Here's how the part is built. I have some questions about the finished solid (model axes, mm). Give positions to 0.01 mm unless a question says otherwise; leave off trailing zeros. Loops run counter-clockwise (first coordinate to the right, second up) from the corner with the lowest first, then second, coordinate; pieces in that order, holes last. Notation, with made-up numbers: (77.25, 30) - (134.25, 30) arc R27 cw to (134.25, 56) - close; hole circle Ø6 at (49.25, 76.25). An arc over 180 degrees is marked (long way). Use a Markdown table: item, result.
Autodesk Inventor part; units mm, degrees
ref_plane "YZ Plane" through (0, 0, 0) normal (1, 0, 0) x (0, 1, 0)
ref_plane "XZ Plane" through (0, 0, 0) normal (0, 1, 0) x (-1, 0, 0)
ref_plane "XY Plane" through (0, 0, 0) normal (0, 0, 1) x (1, 0, 0)
sketch "Sketch1" plane through (0, 0, 0) normal (0, 0, 1) x (1, 0, 0)
  line L0 (0, 0) -> (49.2125, 0)
  arc A0 (69.2791, -9.8278) -> (49.2125, 0) centre (49.2125, -25.4) ccw
  line L1 (69.2791, -9.8278) -> (116.6499, -70.8709)
  arc A1 (113.4684, -97.4512) -> (116.6499, -70.8709) centre (101.6, -82.55) ccw
  line L2 (113.4684, -97.4512) -> (70.102, -131.9913)
  arc A2 (48.0501, -139.7) -> (70.102, -131.9913) centre (48.0501, -104.3043) ccw
  line L3 (48.0501, -139.7) -> (0, -139.7)
  line L4 (0, -139.7) -> (0, 0)
  line L5 (0, -139.7) -> (12.7, -139.7) construction
  circle A3 centre (101.6, -82.55) radius 16 construction
  circle A4 centre (48.0501, -104.3043) radius 7.025 construction
  arc A5 (33.057, -35.4) -> (32.0953, -33.6463) centre (49.2125, -25.4) ccw construction
  circle A6 centre (38.1, -63.5) radius 17.907 construction
  circle A7 centre (71.7198, -40.8503) radius 7.025 construction
  circle A8 centre (38.1, -63.5) radius 19.05
  circle A9 centre (48.0501, -104.3043) radius 3
  circle A10 centre (101.6, -82.55) radius 9.525
  dimension "d0" = 19.05
  dimension "d1" = 38.1
  dimension "d4" = 6
  dimension "d5" = 19.05
extrude "Extrusion1" add sketch "Sketch1" along normal blind 6.35 contours L0 A0 L1 A1 L2 A2 L3 L4 | A8
chamfer "Chamfer1" distance 3.175 angle 45 7 edges at (92.9645, -40.3494, 6.35) (60.3845, -2.5889, 6.35) (24.6062, 0, 6.35) (120.515, -84.8141, 6.35) (91.7852, -114.7212, 6.35) (59.7304, -137.7173, 6.35) (24.0251, -139.7, 6.35)
properties part number "baseOuter" material "Aluminum 6061"
(1) Suppose I cut it at A-A on z = 4.5. Count the separate pieces of the cut face and the enclosed holes in it, plus the area to 3 significant figures.
A:
| item | result |
|---|---|
| separate pieces | 1 |
| enclosed holes | 2 |
| area | 12,400 mm2 |
(2) If I drill on line 1 (Y direction, x = 50, z = 2.5); line 2 (X direction, y = -99, z = 3); line 3 (Y direction, x = 108, z = 5.5), over which ranges is the centre line in solid material (lowest first)?
A:
| item | result |
|---|---|
| line 1 | -139.65 to -106.58, -102.02 to -0.01 |
| line 2 | 0 to 111.52 |
| line 3 | -98.83 to -89.6, -75.5 to -63.52 |
(3) Suppose I cut it at B-B on x = 101.6. Write out the boundary of the cut face in (y, z) (3 decimals), plus the area to 3 significant figures.
A:
| item | result |
|---|---|
| outline | (-106.904, 0) - (-92.075, 0) - (-92.075, 6.35) - (-102.845, 6.35) - (-106.904, 3.175) - close; (-73.025, 0) - (-51.477, 0) - (-51.477, 3.175) - (-56.656, 6.35) - (-73.025, 6.35) - close |
| area | 216 mm2 |
(4) We'd pull the mould along X, two halves only. Please class faces 1 (the face through (94.041, -76.754, 3.131)), 2 (the face through (47.66, -107.28, 3.13)), 3 (the face through (46, -69, 0)), 4 (the face through (0, -71, 3)): pulls with the +X half, pulls with the -X half, needs draft (parallel to the pull), parting line crosses it, or undercut.
A:
| item | result |
|---|---|
| face 1 | undercut |
| face 2 | undercut |
| face 3 | needs draft |
| face 4 | pulls with the -X half |
(5) Suppose I cut it at C-C on y = -112.5. Write out the boundary of the cut face in (x, z) (3 decimals), plus the area to 3 significant figures.
A:
| item | result |
|---|---|
| outline | (0, 0) - (94.574, 0) - (94.574, 3.175) - (89.478, 6.35) - (0, 6.35) - close |
| area | 592 mm2 |
(6) Will these pins go through, and if not, where does the flat tip stop? pin 1 (3 mm diameter, centred on y = -21.5, z = 2, fed in from -X); pin 2 (2 mm diameter, centred on x = 95.5, z = 3.5, fed in from -Y).
A:
| item | result |
|---|---|
| pin 1 | x = 0 |
| pin 2 | y = -112.52 |
(7) Suppose I cut it at D-D on x = 79.5. Write out the boundary of the cut face in (y, z) (3 decimals), plus the area to 3 significant figures.
A:
| item | result |
|---|---|
| outline | (-124.506, 0) - (-22.999, 0) - (-22.999, 3.175) - (-28.177, 6.35) - (-120.447, 6.35) - (-124.506, 3.175) - close |
| area | 630 mm2 |
